```python
from build123d import *

# Parameters (mm, degrees)
SKETCH1_W           = 63.5
SKETCH1_H           = 63.5
SKETCH1_R           = 13.49375
SKETCH1_W_2         = 6.35
SKETCH1_H_2         = 19.05
BOSS_EXTRUDE1_DEPTH = 4.7625


with BuildPart() as part:
    # Sketch1 → Boss-Extrude1 (new body)
    with BuildSketch(Plane.XY):
        with Locations((31.75, 31.75)):
            Rectangle(SKETCH1_W, SKETCH1_H)
        with Locations((31.75, 31.75)):
            Circle(SKETCH1_R, mode=Mode.SUBTRACT)
        with Locations((-3.175, 31.75)):
            Rectangle(SKETCH1_W_2, SKETCH1_H_2)
        with Locations((66.675, 31.75)):
            Rectangle(SKETCH1_W_2, SKETCH1_H_2)
    extrude(amount=BOSS_EXTRUDE1_DEPTH)


solid = part.part
```
Could you check a few things on this model? Use its own coordinates, in mm. A direction names the side the tool comes from. Coordinates: 2 decimals unless noted, no trailing zeros. Order: outer loops, then holes, each group sorted by start corner. A loop starts at its lowest first (then second) coordinate and runs counter-clockwise, first axis right, second up. Notation, with made-up numbers: M -25,82 L 5,82 A17 ccw 5,96 Z; hole C -24,-20 d8. An arc over 180 degrees is marked long. Use one line per item in the form item = value. Start each with the question number.
1. Suppose I cut it at B-B on x = 31.75. Write out the boundary of the cut face in (y, z), then the cut area to 3 significant figures.
2. Please list where these lines run through material, in increasing order: line 1 (Y direction, x = 31.75, z = 3.4); line 2 (X direction, y = 17.5, z = 1.4); line 3 (Y direction, x = 30, z = 3.4).
3. Suppose I cut it at D-D on x = 65.5. Write out the boundary of the cut face in (y, z) (1 decimal).
4. Suppose I cut it at A-A on y = 31.75. Write out the boundary of the cut face in (x, z).
5. For pin 1 (2.5 mm diameter, centred on y = 8.5, z = 2.5, fed in from +X); pin 2 (1.4 mm diameter, centred on x = -4.5, z = 3, fed in from +Y) (3 decimals); pin 3 (2.5 mm diameter, centred on y = 15.5, z = 3.5, fed in from -X), each with a flat end and sliding along its axis, tell me the tip position at first contact or that it passes through.
6. We'd pull the mould along Y, two halves only. Please class faces 1 (the flat face through (-3, 41.275, 2)), 2 (the flat face through (63.5, 11, 2)), 3 (the flat face through (67, 22.225, 2)), 4 (the cylindrical face through (18.27, 32.34, 2.35)): +Y half, -Y half, draft (parallel to the pull), parting line (faces both ways), or undercut.
7. On a 3-axis mill with a long thin cutter (end or side, diameter ignored), from which of +Z, -Z, +X, -X, +Y, -Y can I reach the whole of each face in a straight line? I mean faces 5 (the flat face through (0, 52, 2)), 6 (the flat face through (67, 41.275, 2)), 7 (the flat face through (0, 11, 2)), 8 (the flat face through (31, 0, 2)). Say none if no direction works.
Geometry says:
q1.outline = M 0,0 L 18.26,0 L 18.26,4.76 L 0,4.76 Z; M 45.24,0 L 63.5,0 L 63.5,4.76 L 45.24,4.76 Z
q1.area = 174 mm^2
q2.line_1 = 0 to 18.26, 45.24 to 63.5
q2.line_2 = 0 to 63.5
q2.line_3 = 0 to 18.37, 45.13 to 63.5
q3.outline = M 22.2,0 L 41.3,0 L 41.3,4.8 L 22.2,4.8 Z
q4.outline = M -6.35,0 L 18.26,0 L 18.26,4.76 L -6.35,4.76 Z; M 45.24,0 L 69.85,0 L 69.85,4.76 L 45.24,4.76 Z
q5.pin_1 = 63.5
q5.pin_2 = 41.275
q5.pin_3 = 0
q6.face_1 = +Y half
q6.face_2 = draft
q6.face_3 = -Y half
q6.face_4 = undercut
q7.face_5 = +Z, -Z, -X, +Y
q7.face_6 = +Z, -Z, +X, +Y
q7.face_7 = +Z, -Z, -X, -Y
q7.face_8 = +Z, -Z, +X, -X, -Y
